from build123d import *

# Parameters (mm, degrees)
SKETCH1_R           = 1.778
BOSS_EXTRUDE1_DEPTH = 1.524
SKETCH2_W           = 19.05
SKETCH2_H           = 1.524
BOSS_EXTRUDE2_DEPTH = 11.7475
SKETCH3_R           = 3.048
CUT_EXTRUDE2_DEPTH  = 13.9446
CUT_EXTRUDE3_DEPTH  = 13.9446
SKETCH5_W           = 45.1485
SKETCH5_H           = 1.524
BOSS_EXTRUDE3_DEPTH = 11.7475
FILLET1_R           = 7.9375
FILLET3_R           = 11.6205
FILLET4_R           = 11.6205
FILLET5_R           = 1.524
FILLET6_R           = 1.524
FILLET7_R           = 7.9375


with BuildPart() as part:
    # Sketch1 → Boss-Extrude1 (new body)
    with BuildSketch(Plane.XY):
        Polygon((27.4955, 11.6205), (36.703, 20.5105), (36.703, 22.0345), (-27.4955, 22.0345), (-27.4955, 7.4295), (-27.4955, -11.6205), (27.4955, -11.6205), align=None)
        with Locations(Location((15.875, 0, 0), (0, 0, 180))):
            Circle(SKETCH1_R, mode=Mode.SUBTRACT)
        with Locations(Location((-15.875, 0, 0), (0, 0, 180))):
            Circle(SKETCH1_R, mode=Mode.SUBTRACT)
    extrude(amount=BOSS_EXTRUDE1_DEPTH)

    # Sketch2 → Boss-Extrude2 (add)
    with BuildSketch(Plane.XY.offset(1.524)):
        with Locations((27.178, 21.2725)):
            Rectangle(SKETCH2_W, SKETCH2_H)
    extrude(amount=BOSS_EXTRUDE2_DEPTH)

    # Sketch3 → Cut-Extrude2 (cut)
    with BuildSketch(Plane.XZ.offset(-20.5105)):
        with Locations((28.7655, 5.334)):
            Circle(SKETCH3_R)
    extrude(amount=-CUT_EXTRUDE2_DEPTH, mode=Mode.SUBTRACT)

    # Sketch4 → Cut-Extrude3 (cut)
    with BuildSketch(Plane(origin=(0, 0, 0), x_dir=(-1, 0, 0), z_dir=(0, 0, -1))):
        with BuildLine():
            Line((-19.8755, 11.6205), (-36.703, 11.6205))
            Line((-36.703, 11.6205), (-36.703, 20.5105))
            Line((-36.703, 20.5105), (-19.8755, 20.5105))
            ThreePointArc((-19.8755, 20.5105), (-18.079448776, 19.766551224), (-17.3355, 17.9705))
            Line((-17.3355, 17.9705), (-17.3355, 14.1605))
            ThreePointArc((-17.3355, 14.1605), (-18.079448776, 12.364448776), (-19.8755, 11.6205))
        make_face()
    extrude(amount=-CUT_EXTRUDE3_DEPTH, mode=Mode.SUBTRACT)

    # Sketch5 → Boss-Extrude3 (add)
    with BuildSketch(Plane.XY.offset(1.524)):
        with Locations((-4.92125, 21.2725)):
            Rectangle(SKETCH5_W, SKETCH5_H)
    extrude(amount=BOSS_EXTRUDE3_DEPTH)

    # Fillet1
    fillet1_edges = [part.edges().sort_by_distance(p)[0] for p in [
        (36.703, 21.2725, 13.2715),
    ]]
    fillet(fillet1_edges, radius=FILLET1_R)

    # Fillet3
    fillet3_edges = [part.edges().sort_by_distance(p)[0] for p in [
        (27.4955, -11.6205, 0.762),
    ]]
    fillet(fillet3_edges, radius=FILLET3_R)

    # Fillet4
    fillet4_edges = [part.edges().sort_by_distance(p)[0] for p in [
        (-27.4955, -11.6205, 0.762),
        (27.4955, 11.6205, 0.762),
    ]]
    fillet(fillet4_edges, radius=FILLET4_R)

    # Fillet5
    fillet5_edges = [part.edges().sort_by_distance(p)[0] for p in [
        (-3.81, 20.5105, 1.524),
    ]]
    fillet(fillet5_edges, radius=FILLET5_R)

    # Fillet6
    fillet6_edges = [part.edges().sort_by_distance(p)[0] for p in [
        (4.60375, 22.0345, 0),
    ]]
    fillet(fillet6_edges, radius=FILLET6_R - 0.0001)  # a hair under: the kernel refuses the full size

    # Fillet7
    fillet7_edges = [part.edges().sort_by_distance(p)[0] for p in [
        (-27.4955, 21.2725, 13.2715),
    ]]
    fillet(fillet7_edges, radius=FILLET7_R)


solid = part.part
Read the model definition and answer for the solid it produces. Units are mm, in the model's axes. A direction names the side the tool comes from. Coordinates: 2 decimals unless noted, no trailing zeros. Order: outer loops, then holes, each group sorted by start corner. A loop starts at its lowest first (then second) coordinate and runs counter-clockwise, first axis right, second up. Notation, with made-up numbers: M 24.5,8.5 L 60.5,8.5 A30 cw 60.5,39.5 Z; hole C 74,79.25 d11. An arc over 180 degrees is marked long. Put each result on its own line as item: value. Start each with the question number.
Item 1: The mould has two halves that part along Y. Classify faces 1 (the face through (-3.478, 20.076, 1.982)), 2 (the face through (17.336, 16, 1)), 3 (the face through (-14.464, 1.082, 0.751)), 4 (the face through (0, 4, 1.524)): +Y half, -Y half, draft (parallel to the pull), parting line (faces both ways), or undercut.
Item 2: Section A-A, the plane x = 13 is taken. Determine the outline of the cut face in (y, z), plus the area to 3 significant figures.
Item 3: Section B-B, the plane z = 7 is taken. Determine the outline of the cut face in (x, y), plus the area to 3 significant figures.
Item 4: Consider probe 1 along Y at (x, z) = (-9.5, 4); probe 2 along Z at (x, y) = (-9, -6); probe 3 along Y at (x, z) = (-23.5, 1.75). Determine where each line is inside the solid, lowest interval first. Write a range as [from, to].
Item 5: Section C-C, the plane y = -2.5 is taken. Determine the outline of the cut face in (x, z).
Item 6: For faces 5 (the face through (4.154, 21.576, 0.435)), 6 (the face through (17.828, 12.658, 0.751)), determine the directions among +Z, -Z, +X, -X, +Y, -Y from which every point of the face is accessible in a straight line to the end or side of a thin tool.
Item 7: Section D-D, the plane x = -21 is taken. Determine the outline of the cut face in (y, z), plus the area to 3 significant figures.
Item 8: Given pin 1 Ø2 at (x, y) = (-15.875, 0) entering from -Z; pin 2 Ø1.5 at (x, y) = (-0.5, -5.5) entering from +Z; pin 3 Ø0.5 at (y, z) = (17, 1) entering from +X; pin 4 Ø0.6 at (y, z) = (0.5, 1) entering from +X, each flat-ended and moving along its own axis, determine where each tip first touches the part or whether it passes through.
Computed:
1. face 1: -Y half
1. face 2: undercut
1. face 3: undercut
1. face 4: draft
2. outline: M -11.62,0 L 20.51,0 A1.52 ccw 22.03,1.52 L 22.03,13.27 L 20.51,13.27 L 20.51,3.05 A1.52 cw 18.99,1.52 L -11.62,1.52 Z
2. area: 69.2 mm2
3. outline: M -27.32,20.51 L 26.21,20.51 L 26.21,22.03 L -27.32,22.03 Z; M 31.32,20.51 L 36.53,20.51 L 36.53,22.03 L 31.32,22.03 Z
3. area: 89.5 mm2
4. probe 1: y = [20.51, 22.03]
4. probe 2: z = [0, 1.52]
4. probe 3: y = [19.79, 22.03]
5. outline: M -27.22,0 L 27.22,0 L 27.22,1.52 L -27.22,1.52 Z
6. face 5: -Z, +X, -X, +Y
6. face 6: +Z, -Z, +X
7. outline: M -10.43,0 L 20.51,0 A1.52 ccw 22.03,1.52 L 22.03,13.14 L 20.51,13.14 L 20.51,3.05 A1.52 cw 18.99,1.52 L -10.43,1.52 Z
7. area: 67.2 mm2
8. pin 1: passes through
8. pin 2: stops at z = 1.52
8. pin 3: stops at x = 17.34
8. pin 4: stops at x = 27.5
